from build123d import *

# Parameters (mm, degrees)
BOSS_EXTRUDE1_DEPTH                     = 54.37886
SKETCH6_R                               = 4.762499997
CUT_EXTRUDE2_DEPTH                      = 83.40211381
CBORE_FOR_M8_HEX_HEAD_BOLT1_D           = 9
CBORE_FOR_M8_HEX_HEAD_BOLT1_CBORE_D     = 16
CBORE_FOR_M8_HEX_HEAD_BOLT1_CBORE_DEPTH = 5.68


with BuildPart() as part:
    # Sketch1 → Boss-Extrude1 (new body)
    with BuildSketch(Plane(origin=(0, 0, 0), x_dir=(1, 0, 0), z_dir=(0, 1, 0))):
        Polygon((42.900367849, 10.966428676), (-1.905000006, 4.537947795), (-1.905000006, -33.845088532), (-1.905000006, -33.965034077), (-0.021561819, -33.694806492), (48.313185258, -26.759945507), (47.411349635, -20.474311688), (14.726053775, -25.163856927), (11.793284329, -4.722975747), (44.478580189, -0.033430507), align=None)
    extrude(amount=BOSS_EXTRUDE1_DEPTH)

    # Sketch6 → Cut-Extrude2 (cut, through all)
    with BuildSketch(Plane(origin=(4.736440692, 0, 33.012148819), x_dir=(0.9898635935767917, 0, -0.1420213579404182), z_dir=(0.1420213579404182, 0, 0.9898635935767917))):
        with Locations((29.417979377, 27.18943)):
            Circle(SKETCH6_R)
        Polygon((44.022979377, 36.71443), (29.071940537, 54.37886), (44.022979377, 54.37886), align=None)
        Polygon((44.022979377, 0), (44.022979377, 17.66443), (29.071940537, 0), align=None)
    extrude(amount=-CUT_EXTRUDE2_DEPTH, mode=Mode.SUBTRACT)

    # CBORE for M8 Hex Head Bolt1 (through all)
    with Locations(Plane(origin=(10.891448706, 0, -1.562658073), x_dir=(-0.1420213579404179, 0, -0.9898635935767918), z_dir=(0.9898635935767918, 0, -0.1420213579404179))):
        with Locations((-16.6751, 39.88943), (-16.6751, 14.48943)):
            CounterBoreHole(CBORE_FOR_M8_HEX_HEAD_BOLT1_D / 2, CBORE_FOR_M8_HEX_HEAD_BOLT1_CBORE_D / 2, CBORE_FOR_M8_HEX_HEAD_BOLT1_CBORE_DEPTH)


solid = part.part
Geometry: final body of the model. Coordinates: model frame, mm. A direction names the side the tool comes from. Round coordinates to 2 decimals unless told otherwise and drop trailing zeros. Loops run counter-clockwise (first coordinate to the right, second up) from the corner with the lowest first, then second, coordinate; pieces in that order, holes last. Notation, with made-up numbers: M 53.5,36.5 L 66.5,36.5 A23 cw 66.5,51.5 Z; hole C -40,17 d1. An arc over 180 degrees is marked long. Put each result on its own line as item: value. Start each with the question number.
(1) Draft query along X for faces 1 (the face through (37.77, 25.37, 25.11)), 2 (the face through (7.148, 11.046, 12.341)), 3 (the face through (12, 0, 12)), 4 (the face through (24.28, 26.81, 2.93)). Return one class per face: +X half, -X half, draft (parallel to the pull), parting line (faces both ways), or undercut.
(2) Section query B-B (x = 16). Return loops of the section in (y, z).
(3) Material intervals for line 1 along Y through (x, z) = (7.5, 11); line 2 along Z through (x, y) = (9.5, 11); line 3 along Z through (x, y) = (18, 23.5), sorted ascending. Write a range as [from, to].
(4) Set-up query: faces 5 (the face through (13.28, 26.81, 15.09)), 6 (the face through (28.22, 22.54, -3.17)). Return all of +Z, -Z, +X, -X, +Y, -Y with unobstructed straight access to the full face (end or side cutting, diameter ignored); none if empty.
(5) Section query A-A (y = 13). Return loops of the section in (x, z) (3 decimals), then the cut area to 3 significant figures.
(6) Contact query for flat-ended pins moving along their axis: pin 1 Ø6 at (x, z) = (42.5, 20) entering from -Y; pin 2 Ø1 at (x, y) = (36.5, 16.5) entering from -Z; pin 3 Ø4 at (x, y) = (14.5, 5.5) entering from -Z. Output: stop coordinate, or through.
(7) Section query C-C (y = 7.5). Return loops of the section in (x, z) (1 decimal).
(8) Section query D-D (z = 13.5). State how many separate pieces and enclosed holes the cut face has, then the cut area to 3 significant figures.
Findings below:
1. face 1: undercut
1. face 2: undercut
1. face 3: draft
1. face 4: +X half
2. outline: M 0,-7.11 L 54.38,-7.11 L 54.38,4.12 L 0,4.12 Z; M 0,24.98 L 54.38,24.98 L 54.38,31.4 L 0,31.4 Z
3. line 1: y = [0, 8.03], [20.95, 33.43], [46.35, 54.38]
3. line 2: z = [-6.17, 8.21], [22.76, 32.33]
3. line 3: z = [-7.39, 3.83], [24.69, 31.11]
4. face 5: +Y, -Y
4. face 6: none
5. outline: M -1.905,-4.538 L 38.992,-10.406 L 40.571,0.594 L 11.793,4.723 L 12.143,7.163 L 6.521,7.97 L 7.034,11.547 L -1.905,12.829 Z; M -1.905,21.409 L 8.24,19.953 L 8.754,23.531 L 14.376,22.724 L 14.726,25.164 L 43.503,21.035 L 44.405,27.321 L -1.905,33.965 Z
5. area: 907 mm2
6. pin 1: stops at y = 8.73
6. pin 2: stops at z = -10.12
6. pin 3: stops at z = -7.18
7. outline: M -1.9,-4.5 L 34.4,-9.7 L 36,1.3 L 11.8,4.7 L 12.7,11.1 L 7.1,11.9 L 8.2,19.6 L 13.8,18.8 L 14.7,25.2 L 38.9,21.7 L 39.8,28 L -1.9,34 Z
8. separate pieces: 3
8. enclosed holes: 0
8. area: 510 mm2
